Could you check a few things on this drawing? It's one solid part, dimensions in mm from its lowest x, y, z. Coordinates: 2 decimals unless noted, no trailing zeros. Write each loop counter-clockwise with the first axis right and the second up, starting at its lowest first coordinate (ties: lowest second). Pieces come first, ordered by that corner, then holes.
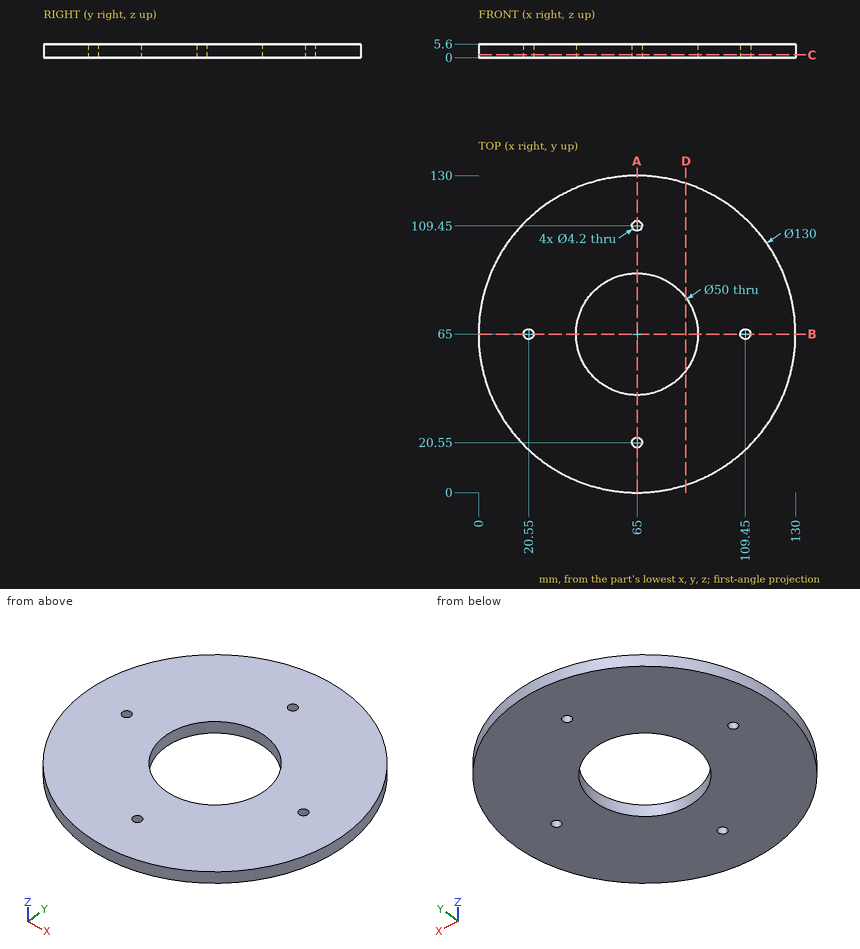
1) Imagine slicing it at A-A on x = 65. Please give me the cut outline in (y, z), then the cut area to 3 significant figures.
Values follow:
outline: (0, 0) - (18.45, 0) - (18.45, 5.6) - (0, 5.6) - close; (22.65, 0) - (40, 0) - (40, 5.6) - (22.65, 5.6) - close; (90, 0) - (107.35, 0) - (107.35, 5.6) - (90, 5.6) - close; (111.55, 0) - (130, 0) - (130, 5.6) - (111.55, 5.6) - close
area: 401 mm2
2) Will these pins go through, and if not, where does the flat tip stop? pin 1 (2 mm diameter, centred on x = 49, z = 2, fed in from -Y); pin 2 (1 mm diameter, centred on x = 94.5, z = 1.5, fed in from -Y); pin 3 (2 mm diameter, centred on y = 33, z = 2.5, fed in from +X).
Values follow:
pin 1: stops at y = 1.75
pin 2: stops at y = 6.83
pin 3: stops at x = 122.13
3) Imagine slicing it at D-D on x = 85. Please give me the cut outline in (y, z).
Values follow:
outline: (3.15, 0) - (50, 0) - (50, 5.6) - (3.15, 5.6) - close; (80, 0) - (126.85, 0) - (126.85, 5.6) - (80, 5.6) - close
4) I need wall thicknesses on probe 1 along X at (y, z) = (65, 3.9); probe 2 along X at (y, z) = (20.55, 4.05); probe 3 along X at (y, z) = (57, 4.55). Which ranges of each line are inside material? Lowest first, please.
Values follow:
probe 1: x = 0 to 18.45, 22.65 to 40, 90 to 107.35, 111.55 to 130
probe 2: x = 17.57 to 62.9, 67.1 to 112.43
probe 3: x = 0.49 to 41.31, 88.69 to 129.51
5) Imagine slicing it at C-C on z = 1.15. Please give me the cut outline in (x, y), then the cut area to 3 significant figures.
Values follow:
outline: circle Ø130 at (65, 65); hole circle Ø4.2 at (20.55, 65); hole circle Ø50 at (65, 65); hole circle Ø4.2 at (65, 20.55); hole circle Ø4.2 at (65, 109.45); hole circle Ø4.2 at (109.45, 65)
area: 11,300 mm2
